Part model, mm, in its own coordinate system. A direction names the side the tool comes from. Round coordinates to 2 decimals unless told otherwise and drop trailing zeros. Loops run counter-clockwise (first coordinate to the right, second up) from the corner with the lowest first, then second, coordinate; pieces in that order, holes last. Notation, with made-up numbers: (85, 66) - (110, 66) arc R21 cw to (110, 82) - close; hole circle Ø4 at (52, -3). An arc over 180 degrees is marked (long way). Put each result on its own line as item: value.
from build123d import *

# Parameters (mm, degrees)
SKETCH1_R           = 18
SKETCH1_R_2         = 9
SKETCH1_R_3         = 2.15
BOSS_EXTRUDE1_DEPTH = 3
BOSS_EXTRUDE2_START = -8
SKETCH2_R           = 18
BOSS_EXTRUDE2_DEPTH = 8


with BuildPart() as part:
    # Sketch1 → Boss-Extrude1 (new body)
    with BuildSketch(Plane(origin=(0, 0, 0), x_dir=(1, 0, 0), z_dir=(0, 1, 0))):
        with Locations(Location((0, 0, 0), (0, 0, 270))):
            Circle(SKETCH1_R)
        with Locations(Location((0, 0, 0), (0, 0, 270))):
            Circle(SKETCH1_R_2, mode=Mode.SUBTRACT)
        with Locations(Location((0, -13.5, 0), (0, 0, 270))):
            Circle(SKETCH1_R_3, mode=Mode.SUBTRACT)
        with Locations(Location((-13.5, 0, 0), (0, 0, 270))):
            Circle(SKETCH1_R_3, mode=Mode.SUBTRACT)
        with Locations(Location((0, 13.5, 0), (0, 0, 270))):
            Circle(SKETCH1_R_3, mode=Mode.SUBTRACT)
        with Locations(Location((13.5, 0, 0), (0, 0, 270))):
            Circle(SKETCH1_R_3, mode=Mode.SUBTRACT)
    extrude(amount=BOSS_EXTRUDE1_DEPTH)

    # Sketch2 → Boss-Extrude2 (add)
    with BuildSketch(Plane(origin=(0, 3, 0), x_dir=(1, 0, 0), z_dir=(0, 1, 0)).offset(BOSS_EXTRUDE2_START)):
        with BuildLine():
            Line((22.477766793, 1), (25.306193918, 0))
            Line((25.306193918, 0), (22.477766793, -1))
            ThreePointArc((22.477766793, -1), (22.409421615, -2.01688445), (22.295096728, -3.029630652))
            Line((22.295096728, -3.029630652), (24.89951297, -4.518595405))
            Line((24.89951297, -4.518595405), (21.937982938, -4.997489829))
            ThreePointArc((21.937982938, -4.997489829), (21.689164366, -5.985829025), (21.39584391, -6.961886482))
            Line((21.39584391, -6.961886482), (23.692541189, -8.891959436))
            Line((23.692541189, -8.891959436), (20.693094262, -8.834356223))
            ThreePointArc((20.693094262, -8.834356223), (20.271799528, -9.76238413), (19.808911064, -10.670381552))
            Line((19.808911064, -10.670381552), (21.724071639, -12.979528574))
            Line((21.724071639, -12.979528574), (18.783112509, -12.387279139))
            ThreePointArc((18.783112509, -12.387279139), (18.202882373, -13.225168177), (17.585303517, -14.03592178))
            Line((17.585303517, -14.03592178), (19.057372553, -16.649924985))
            Line((19.057372553, -16.649924985), (16.269426065, -15.542064712))
            ThreePointArc((16.269426065, -15.542064712), (15.548909602, -16.262884436), (14.796489846, -16.950335932))
            Line((14.796489846, -16.950335932), (15.778153832, -19.785179106))
            Line((15.778153832, -19.785179106), (13.232826882, -18.197315536))
            ThreePointArc((13.232826882, -18.197315536), (12.395182083, -18.777898209), (11.532104817, -19.319952342))
            Line((11.532104817, -19.319952342), (11.991812264, -22.284521292))
            Line((11.991812264, -22.284521292), (9.770913754, -20.267689666))
            ThreePointArc((9.770913754, -20.267689666), (8.843063212, -20.689374882), (7.897068451, -21.068609586))
            Line((7.897068451, -21.068609586), (7.820043984, -24.067620628))
            Line((7.820043984, -24.067620628), (5.994955418, -21.686643575))
            ThreePointArc((5.994955418, -21.686643575), (5.006721014, -21.935878024), (4.008213807, -22.140104383))
            Line((4.008213807, -22.140104383), (3.396933055, -25.077166834))
            Line((3.396933055, -25.077166834), (2.026314283, -22.408570914))
            ThreePointArc((2.026314283, -22.408570914), (1.009458683, -22.477343997), (-0.009468127, -22.499998008))
            Line((-0.009468127, -22.499998008), (-1.135358097, -25.280712264))
            Line((-1.135358097, -25.280712264), (-2.00745426, -22.410268347))
            ThreePointArc((-2.00745426, -22.410268347), (-3.020248481, -22.29636964), (-4.026845748, -22.136723184))
            Line((-4.026845748, -22.136723184), (-5.631157905, -24.671714801))
            Line((-5.631157905, -24.671714801), (-5.976701572, -21.691681316))
            ThreePointArc((-5.976701572, -21.691681316), (-6.952882373, -21.398771617), (-7.914797233, -21.061955863))
            Line((-7.914797233, -21.061955863), (-9.945967666, -23.269748125))
            Line((-9.945967666, -23.269748125), (-9.753852778, -20.275905799))
            ThreePointArc((-9.753852778, -20.275905799), (-10.662044906, -19.813399467), (-11.548360622, -19.31023995))
            Line((-11.548360622, -19.31023995), (-13.941105841, -21.119872597))
            Line((-13.941105841, -21.119872597), (-13.21750713, -18.208445987))
            ThreePointArc((-13.21750713, -18.208445987), (-14.028520542, -17.591208356), (-14.810750199, -16.937877037))
            Line((-14.810750199, -16.937877037), (-17.488165405, -18.291186987))
            Line((-17.488165405, -18.291186987), (-16.256339927, -15.555751739))
            ThreePointArc((-16.256339927, -15.555751739), (-16.944107985, -14.803621334), (-17.597110079, -14.02111682))
            Line((-17.597110079, -14.02111682), (-20.473140942, -14.874607576))
            Line((-20.473140942, -14.874607576), (-18.772680583, -12.403082831))
            ThreePointArc((-18.772680583, -12.403082831), (-19.315097856, -11.540233742), (-19.817884361, -10.653706371))
            Line((-19.817884361, -10.653706371), (-22.800092885, -10.97994604))
            Line((-22.800092885, -10.97994604), (-20.68565184, -8.851768635))
            ThreePointArc((-20.68565184, -8.851768635), (-21.065284589, -7.905933542), (-21.401695534, -6.943877034))
            Line((-21.401695534, -6.943877034), (-24.394231082, -6.732380003))
            Line((-24.394231082, -6.732380003), (-21.933769225, -5.015951312))
            ThreePointArc((-21.933769225, -5.015951312), (-22.138415743, -4.017530133), (-22.297638603, -3.010865775))
            Line((-22.297638603, -3.010865775), (-25.204318621, -2.268429734))
            Line((-25.204318621, -2.268429734), (-22.476917221, -1.018917187))
            ThreePointArc((-22.476917221, -1.018917187), (-22.5, 0), (-22.476917221, 1.018917187))
            Line((-22.476917221, 1.018917187), (-25.204318621, 2.268429734))
            Line((-25.204318621, 2.268429734), (-22.297638603, 3.010865775))
            ThreePointArc((-22.297638603, 3.010865775), (-22.138415743, 4.017530133), (-21.933769225, 5.015951312))
            Line((-21.933769225, 5.015951312), (-24.394231082, 6.732380003))
            Line((-24.394231082, 6.732380003), (-21.401695534, 6.943877034))
            ThreePointArc((-21.401695534, 6.943877034), (-21.065284589, 7.905933542), (-20.68565184, 8.851768635))
            Line((-20.68565184, 8.851768635), (-22.800092885, 10.97994604))
            Line((-22.800092885, 10.97994604), (-19.817884361, 10.653706371))
            ThreePointArc((-19.817884361, 10.653706371), (-19.315097856, 11.540233742), (-18.772680583, 12.403082831))
            Line((-18.772680583, 12.403082831), (-20.473140942, 14.874607576))
            Line((-20.473140942, 14.874607576), (-17.597110079, 14.02111682))
            ThreePointArc((-17.597110079, 14.02111682), (-16.944107985, 14.803621334), (-16.256339927, 15.555751739))
            Line((-16.256339927, 15.555751739), (-17.488165405, 18.291186987))
            Line((-17.488165405, 18.291186987), (-14.810750199, 16.937877037))
            ThreePointArc((-14.810750199, 16.937877037), (-14.028520542, 17.591208356), (-13.21750713, 18.208445987))
            Line((-13.21750713, 18.208445987), (-13.941105841, 21.119872597))
            Line((-13.941105841, 21.119872597), (-11.548360622, 19.31023995))
            ThreePointArc((-11.548360622, 19.31023995), (-10.662044906, 19.813399467), (-9.753852778, 20.275905799))
            Line((-9.753852778, 20.275905799), (-9.945967666, 23.269748125))
            Line((-9.945967666, 23.269748125), (-7.914797233, 21.061955863))
            ThreePointArc((-7.914797233, 21.061955863), (-6.952882373, 21.398771617), (-5.976701572, 21.691681316))
            Line((-5.976701572, 21.691681316), (-5.631157905, 24.671714801))
            Line((-5.631157905, 24.671714801), (-4.026845748, 22.136723184))
            ThreePointArc((-4.026845748, 22.136723184), (-3.020248481, 22.29636964), (-2.00745426, 22.410268347))
            Line((-2.00745426, 22.410268347), (-1.135358097, 25.280712264))
            Line((-1.135358097, 25.280712264), (-0.009468127, 22.499998008))
            ThreePointArc((-0.009468127, 22.499998008), (1.009458683, 22.477343997), (2.026314283, 22.408570914))
            Line((2.026314283, 22.408570914), (3.396933055, 25.077166834))
            Line((3.396933055, 25.077166834), (4.008213807, 22.140104383))
            ThreePointArc((4.008213807, 22.140104383), (5.006721014, 21.935878024), (5.994955418, 21.686643575))
            Line((5.994955418, 21.686643575), (7.820043984, 24.067620628))
            Line((7.820043984, 24.067620628), (7.897068451, 21.068609586))
            ThreePointArc((7.897068451, 21.068609586), (8.843063212, 20.689374882), (9.770913754, 20.267689666))
            Line((9.770913754, 20.267689666), (11.991812264, 22.284521292))
            Line((11.991812264, 22.284521292), (11.532104817, 19.319952342))
            ThreePointArc((11.532104817, 19.319952342), (12.395182083, 18.777898209), (13.232826882, 18.197315536))
            Line((13.232826882, 18.197315536), (15.778153832, 19.785179106))
            Line((15.778153832, 19.785179106), (14.796489846, 16.950335932))
            ThreePointArc((14.796489846, 16.950335932), (15.548909602, 16.262884436), (16.269426065, 15.542064712))
            Line((16.269426065, 15.542064712), (19.057372553, 16.649924985))
            Line((19.057372553, 16.649924985), (17.585303517, 14.03592178))
            ThreePointArc((17.585303517, 14.03592178), (18.202882373, 13.225168177), (18.783112509, 12.387279139))
            Line((18.783112509, 12.387279139), (21.724071639, 12.979528574))
            Line((21.724071639, 12.979528574), (19.808911064, 10.670381552))
            ThreePointArc((19.808911064, 10.670381552), (20.271799528, 9.76238413), (20.693094262, 8.834356223))
            Line((20.693094262, 8.834356223), (23.692541189, 8.891959436))
            Line((23.692541189, 8.891959436), (21.39584391, 6.961886482))
            ThreePointArc((21.39584391, 6.961886482), (21.689164366, 5.985829025), (21.937982938, 4.997489829))
            Line((21.937982938, 4.997489829), (24.89951297, 4.518595405))
            Line((24.89951297, 4.518595405), (22.295096728, 3.029630652))
            ThreePointArc((22.295096728, 3.029630652), (22.409421615, 2.01688445), (22.477766793, 1))
        make_face()
        with Locations(Location((0, 0, 0), (0, 0, 270))):
            Circle(SKETCH2_R, mode=Mode.SUBTRACT)
    extrude(amount=BOSS_EXTRUDE2_DEPTH)


solid = part.part
1. Pin check, flat tips, straight feed: P1, Ø1, axis at x = 6.5, y = -2.5, coming from the +Z side; P2, Ø4, axis at x = 0, z = 13.5, coming from the +Y side; P3, Ø5, axis at x = 0, z = -13.5, coming from the -Y side; P4, Ø3, axis at x = 1, y = -2.5, coming from the +Z side. Stop position of each tip, or through.
A:
P1: stops at z = 23
P2: passes through
P3: stops at y = 0
P4: stops at z = 23.71
2. Two-plate mould, pull along X, no slides. Class faces 1 (the flat face through (17.683, -1.056, 16.104)), 2 (the flat face through (-21.758, -1.056, 9.931)), 3 (the flat face through (-11, 3, 0)): pulls with the +X half, pulls with the -X half, needs draft (parallel to the pull), parting line crosses it, or undercut.
A:
face 1: undercut
face 2: pulls with the -X half
face 3: needs draft
3. Tool access for faces 4 (the cylindrical face through (-19.31, -1.06, 11.55)), 5 (the flat face through (-16.86, -1.06, -16.9)), 6 (the flat face through (2.72, -1.06, 23.76)), 7 (the flat face through (-19.055, -1.056, -14.454)): list every direction of +Z, -Z, +X, -X, +Y, -Y with a clear straight run to the whole face (end or side of a thin tool).
A:
face 4: +Y, -Y
face 5: -X, +Y, -Y
face 6: +Z, +Y, -Y
face 7: -Z, +Y, -Y
4. Band-saw the part on B-B (y = 1). Give the number of separate pieces and of enclosed holes in the cut face, plus the area to 3 significant figures.
A:
separate pieces: 1
enclosed holes: 5
area: 1,380 mm²
5. Band-saw the part on A-A (z = -8). List the corners of the cut face in (x, y), plus the area to 3 significant figures.
A:
outline: (-21.03, -5) - (-16.12, -5) - (-16.12, 0) - (-4.12, 0) - (-4.12, 3) - (-21.03, 3) - close; (4.12, 0) - (16.12, 0) - (16.12, -5) - (22.63, -5) - (22.63, 3) - (4.12, 3) - close
area: 163 mm²
6. Probe line 1 along X through (y, z) = (2.5, 20.5); line 2 along Y through (x, z) = (-14, 11); line 3 along X through (y, z) = (1.8, 13.5). List the from-to ranges inside material, lowest first. Write a range as [from, to].
A:
line 1: x = [-13.79, -13.12], [-9.77, 9.27], [10.03, 11.72]
line 2: y = [0, 3]
line 3: x = [-19.53, -2.15], [2.15, 18]
